```python
from build123d import *

# Parameters (mm, degrees)
SKETCH1_R           = 2.5
BOSS_EXTRUDE1_DEPTH = 6
SKETCH2_R           = 15
BOSS_EXTRUDE2_DEPTH = 2
BOSS_EXTRUDE3_START = 2
SKETCH3_R           = 15
BOSS_EXTRUDE3_DEPTH = 2
FILLET9_R           = 3
FILLET10_R          = 3
SKETCH4_R           = 1.5
CUT_EXTRUDE1_DEPTH  = 10
SKETCH5_R           = 1.999371682
CUT_EXTRUDE2_DEPTH  = 0.7
SKETCH7_R           = 0.8
CUT_EXTRUDE6_DEPTH  = 3


with BuildPart() as part:
    # Sketch1 → Boss-Extrude1 (new body)
    with BuildSketch(Plane.XY):
        Circle(SKETCH1_R)
    extrude(amount=BOSS_EXTRUDE1_DEPTH)

    # Sketch2 → Boss-Extrude2 (add)
    with BuildSketch(Plane(origin=(0, 0, 0), x_dir=(-1, 0, 0), z_dir=(0, 0, -1))):
        Circle(SKETCH2_R)
    extrude(amount=BOSS_EXTRUDE2_DEPTH)

    # Sketch3 → Boss-Extrude3 (add)
    with BuildSketch(Plane.XY.offset(6).offset(BOSS_EXTRUDE3_START)):
        with Locations(Location((0, 0, 0), (0, 0, 180))):
            Circle(SKETCH3_R)
    extrude(amount=-BOSS_EXTRUDE3_DEPTH)

    # Fillet9
    fillet9_edges = [part.edges().sort_by_distance(p)[0] for p in [
        (-2.5, 0, 0),
    ]]
    fillet(fillet9_edges, radius=FILLET9_R)

    # Fillet10
    fillet10_edges = [part.edges().sort_by_distance(p)[0] for p in [
        (-2.5, 0, 6),
    ]]
    fillet(fillet10_edges, radius=FILLET10_R - 0.0001)  # a hair under: the kernel refuses the full size

    # Sketch4 → Cut-Extrude1 (cut)
    with BuildSketch(Plane(origin=(0, 0, -2), x_dir=(-1, 0, 0), z_dir=(0, 0, -1))):
        Circle(SKETCH4_R)
    extrude(amount=-CUT_EXTRUDE1_DEPTH, mode=Mode.SUBTRACT)

    # Sketch5 → Cut-Extrude2 (cut)
    with BuildSketch(Plane.XY.offset(8)):
        Circle(SKETCH5_R)
    extrude(amount=-CUT_EXTRUDE2_DEPTH, mode=Mode.SUBTRACT)

    # Sketch7 → Cut-Extrude6 (cut)
    with BuildSketch(Plane.XY.offset(8)):
        with Locations((4.509371682, 0)):
            Circle(SKETCH7_R)
        with Locations((-4.509371682, 0)):
            Circle(SKETCH7_R)
    extrude(amount=-CUT_EXTRUDE6_DEPTH, mode=Mode.SUBTRACT)


solid = part.part
```
Verification items for the finished model (mm, model axes). A direction names the side the tool comes from. Give positions to 0.01 mm unless a question says otherwise; leave off trailing zeros. Order: outer loops, then holes, each group sorted by start corner. A loop starts at its lowest first (then second) coordinate and runs counter-clockwise, first axis right, second up. Notation, with made-up numbers: M 39.5,-15 L 98.5,-15 A24 cw 98.5,-3 Z; hole C -21.75,-9 d4. An arc over 180 degrees is marked long. Answer in a Markdown table with one row per item. Add a question column.
Item 1: Section check D-D, the plane y = 13.25. Enter the section's corners in (x, z).
Item 2: Section check C-C, the plane z = -0.75. Enter the section's corners in (x, y), and give its area (3 significant figures).
Item 3: Tool access check on faces 1 (the cylindrical face through (-3.746, 0.24, 7.01)), 2 (the cylindrical face through (-8.06, -12.65, 7.01)), 3 (the flat face through (-6, 0, 0)). Record the directions out of +Z, -Z, +X, -X, +Y, -Y that give a thin tool (end or side, any length) a straight path to the whole face; none if there is none.
Item 4: Gauge pin test, flat ends, axial feed: pin 1 (1.3 mm diameter, centred on x = -4.51, y = 0, fed in from +Z); pin 2 (1 mm diameter, centred on x = -9, z = 1.5, fed in from -Y); pin 3 (5 mm diameter, centred on y = 6.5, z = 4.5, fed in from -X). Record the tip position at first contact, or that the pin passes through.
Item 5: Section check B-B, the plane y = -10.5. Enter the section's corners in (x, z).
Item 6: Scan lines: probe 1 along Z at (x, y) = (-7.75, -5.5); probe 2 along X at (y, z) = (-0.25, 7); probe 3 along X at (y, z) = (1, 3). Record each from-to range of solid material in increasing order. Write a range as from..to.
Item 7: Mould release check, pull along X, two halves, no side actions. Record for faces 4 (the flat face through (-6, 0, 6)), 5 (the cylindrical face through (14.985, 0.66, -0.986)), 6 (the cylindrical face through (3.71, 0.04, 7.01)): released by +X, released by -X, zero draft, split by the parting line, or undercut.
Filled sheet:
| question | item | result |
|---|---|---|
| 1 | outline | M -7.03,-2 L 7.03,-2 L 7.03,0 L -7.03,0 Z; M -7.03,6 L 7.03,6 L 7.03,8 L -7.03,8 Z |
| 2 | outline | C 0,0 d30; hole C 0,0 d3 |
| 2 | area | 700 mm^2 |
| 3 | face 1 | +Z |
| 3 | face 2 | +Z, -Z |
| 3 | face 3 | none |
| 4 | pin 1 | stops at z = 0.49 |
| 4 | pin 2 | passes through |
| 4 | pin 3 | stops at x = -14.31 |
| 5 | outline | M -10.71,-2 L 10.71,-2 L 10.71,0 L -10.71,0 Z; M -10.71,6 L 10.71,6 L 10.71,8 L -10.71,8 Z |
| 6 | probe 1 | z = -2..0, 6..8 |
| 6 | probe 2 | x = -15..-5.27, -3.75..-1.48, 1.48..3.75, 5.27..15 |
| 6 | probe 3 | x = -2.29..-1.12, 1.12..2.29 |
| 7 | face 4 | zero draft |
| 7 | face 5 | split by the parting line |
| 7 | face 6 | undercut |
